from build123d import *

# Parameters (mm, degrees)
SKETCH1_W           = 25
SKETCH1_H           = 22
SKETCH1_R           = 1
SKETCH1_R_2         = 5
BOSS_EXTRUDE1_DEPTH = 3
SKETCH2_W           = 40
SKETCH2_H           = 8
BOSS_EXTRUDE2_DEPTH = 25
CHAMFER1_SIZE       = 7
SKETCH3_W           = 40
SKETCH3_H           = 2
CUT_EXTRUDE1_DEPTH  = 25
SKETCH7_W           = 21
SKETCH7_H           = 12
CUT_EXTRUDE2_DEPTH  = 3
SKETCH8_W           = 15
SKETCH8_H           = 12
CUT_EXTRUDE3_DEPTH  = 31
SKETCH9_R           = 1.25
CUT_EXTRUDE4_DEPTH  = 31
BOSS_EXTRUDE3_START = -3
BOSS_EXTRUDE3_DEPTH = 3
SKETCH11_R          = 1
CUT_EXTRUDE5_DEPTH  = 3


with BuildPart() as part:
    # Sketch1 → Boss-Extrude1 (new body)
    with BuildSketch(Plane(origin=(0, 0, 0), x_dir=(1, 0, 0), z_dir=(0, 1, 0))):
        Rectangle(SKETCH1_W, SKETCH1_H)
        with Locations((6, 8)):
            Circle(SKETCH1_R, mode=Mode.SUBTRACT)
        with Locations((-6, 8)):
            Circle(SKETCH1_R, mode=Mode.SUBTRACT)
        Circle(SKETCH1_R_2, mode=Mode.SUBTRACT)
        with Locations((-8.5, -6)):
            Circle(SKETCH1_R, mode=Mode.SUBTRACT)
        with Locations((8.5, -6)):
            Circle(SKETCH1_R, mode=Mode.SUBTRACT)
    extrude(amount=BOSS_EXTRUDE1_DEPTH)

    # Sketch2 → Boss-Extrude2 (add)
    with BuildSketch(Plane(origin=(0, 3, 0), x_dir=(1, 0, 0), z_dir=(0, 1, 0))):
        Rectangle(SKETCH2_W, SKETCH2_H)
    extrude(amount=BOSS_EXTRUDE2_DEPTH)

    # Chamfer1
    chamfer1_edges = [part.edges().sort_by_distance(p)[0] for p in [
        (20, 3, 0),
        (-20, 3, 0),
    ]]
    chamfer(chamfer1_edges, length=CHAMFER1_SIZE)

    # Sketch3 → Cut-Extrude1 (cut)
    with BuildSketch(Plane(origin=(0, 28, 0), x_dir=(1, 0, 0), z_dir=(0, 1, 0))):
        Rectangle(SKETCH3_W, SKETCH3_H)
    extrude(amount=-CUT_EXTRUDE1_DEPTH, mode=Mode.SUBTRACT)

    # Sketch7 → Cut-Extrude2 (cut)
    with BuildSketch(Plane.XY.offset(4)):
        with Locations((7, 19)):
            Rectangle(SKETCH7_W, SKETCH7_H)
    extrude(amount=-CUT_EXTRUDE2_DEPTH, mode=Mode.SUBTRACT)

    # Sketch8 → Cut-Extrude3 (cut)
    with BuildSketch(Plane.XY.offset(-1)):
        with Locations((10, 19)):
            Rectangle(SKETCH8_W, SKETCH8_H)
    extrude(amount=-CUT_EXTRUDE3_DEPTH, mode=Mode.SUBTRACT)

    # Sketch9 → Cut-Extrude4 (cut)
    with BuildSketch(Plane.XY.offset(4)):
        with Locations((-12.5, 19)):
            Circle(SKETCH9_R)
    extrude(amount=-CUT_EXTRUDE4_DEPTH, mode=Mode.SUBTRACT)

    # Sketch10 → Boss-Extrude3 (add)
    with BuildSketch(Plane.XY.offset(4).offset(BOSS_EXTRUDE3_START)):
        Polygon((20, 10), (22.5, 12.5), (22.5, 28), (20, 28), align=None)
    extrude(amount=BOSS_EXTRUDE3_DEPTH)

    # Sketch11 → Cut-Extrude5 (cut)
    with BuildSketch(Plane.XY.offset(4)):
        with Locations((20.5, 19.311850015)):
            Circle(SKETCH11_R)
        with Locations((-6.5, 19.311850015)):
            Circle(SKETCH11_R)
    extrude(amount=-CUT_EXTRUDE5_DEPTH, mode=Mode.SUBTRACT)


solid = part.part
Build history of the part. All positions in model axes, mm. A direction names the side the tool comes from. Round coordinates to 2 decimals unless told otherwise and drop trailing zeros. Loops run counter-clockwise (first coordinate to the right, second up) from the corner with the lowest first, then second, coordinate; pieces in that order, holes last. Notation, with made-up numbers: (-32.75, 34) -> (12.25, 34) arc R19 ccw to (12.25, 66) -> close; hole circle Ø8 at (89.25, -0.5). An arc over 180 degrees is marked (long way). Use CSV: the item, a comma, the result in double quotes. Start each with the question number.
Q1. Flat gauge pins, fed straight in: pin 1 Ø3.5 at (y, z) = (1.5, -2.5) entering from -X; pin 2 Ø1.6 at (x, y) = (-6.5, 19.31) entering from -Z; pin 3 Ø2.5 at (x, z) = (-6, -8) entering from +Y. Where does each tip first touch, or does it go through?
Q2. Mould opens along Z. For faces 1 (the face through (0, 1, 11)), 2 (the face through (16, 6, -2)), 3 (the face through (0, 3, -3)) say: +Z half, -Z half, draft (parallel to the pull), parting line (faces both ways), or undercut.
Q3. Saw through at C-C on y = 24. Give the cut face in (x, z), and give its area (4 significant figures).
Q4. Which spindle directions (+Z, -Z, +X, -X, +Y, -Y) get a long thin tool onto all of the face, cutting with end or side? Do faces 4 (the face through (17.5, 19, 3)), 5 (the face through (20, 19, -2)), 6 (the face through (0, 3, 2)), 7 (the face through (-12.5, 1, 0)), 8 (the face through (-4, 16, 4)). Say none if no direction does.
Q5. Saw through at A-A on z = 0. Give the cut face in (x, y).
Q6. Saw through at D-D on x = 6. Give the cut face in (y, z).
Q7. Saw through at B-B on x = 18. Give the cut face in (y, z), and give its area (3 significant figures).
Q8. Drill centre lines: L1, parallel to X at y = 1.4, z = -8; L2, parallel to X at y = 0.65, z = 6; L3, parallel to Y at x = 8, z = -2.25. Where is each one in solid material? Low to high.
Solutions:
1,pin 1,"stops at x = -13.25"
1,pin 2,"stops at z = -4"
1,pin 3,"stops at y = 3"
2,face 1,"+Z half"
2,face 2,"draft"
2,face 3,"undercut"
3,outline,"(-20, -4) -> (2.5, -4) -> (2.5, -1) -> (-20, -1) -> close; (-20, 1) -> (-3.5, 1) -> (-3.5, 4) -> (-20, 4) -> close; (17.5, -4) -> (20, -4) -> (20, -1) -> (17.5, -1) -> close; (17.5, 1) -> (22.5, 1) -> (22.5, 4) -> (17.5, 4) -> close"
3,area,"139.5 mm^2"
4,face 4,"+Z, -Z"
4,face 5,"-Z, +X, +Y, -Y"
4,face 6,"-Y"
4,face 7,"+Z, -Z, -X, -Y"
4,face 8,"+Z, +X, -X, +Y"
5,outline,"(-12.5, 0) -> (-5, 0) -> (-5, 3) -> (-12.5, 3) -> close; (5, 0) -> (12.5, 0) -> (12.5, 3) -> (5, 3) -> close"
6,outline,"(0, -11) -> (3, -11) -> (3, -9) -> (0, -9) -> close; (0, -7) -> (3, -7) -> (3, -4) -> (13, -4) -> (13, -1) -> (3, -1) -> (3, 1) -> (13, 1) -> (13, 4) -> (3, 4) -> (3, 11) -> (0, 11) -> close; (25, -4) -> (28, -4) -> (28, -1) -> (25, -1) -> close; (25, 1) -> (28, 1) -> (28, 4) -> (25, 4) -> close"
7,outline,"(8, -4) -> (28, -4) -> (28, -1) -> (8, -1) -> close; (8, 1) -> (28, 1) -> (28, 4) -> (8, 4) -> close"
7,area,"120 mm^2"
8,L1,"x = -12.5 to -7, -5 to 5, 7 to 12.5"
8,L2,"x = -12.5 to -9.5, -7.5 to 7.5, 9.5 to 12.5"
8,L3,"y = 0 to 13, 25 to 28"
